```python
from build123d import *

# Parameters (mm, degrees)
F1_DEPTH = 120
F2_T     = -2
F3_W     = 48
F3_H     = 27.5
F4_DEPTH = 3


with BuildPart() as f1:
    # F0 (on Right) → F1 (new body)
    with BuildSketch(Plane.YZ):
        Polygon((0, 0), (0, 52), (-55, 52), (-94, 22), (-94, 0), align=None)
    extrude(amount=F1_DEPTH)

    # F2
    f2_openings = [f1.faces().sort_by_distance(p)[0] for p in [
        (60, -27.5, 52),
    ]]
    offset(amount=F2_T, openings=f2_openings, kind=Kind.INTERSECTION)

    # F3 (on face) → F4 (cut)
    with BuildSketch(Plane(origin=(0, -45.5762081784, 59.249070632), x_dir=(1, 0, 0), z_dir=(0, -0.6097107608, 0.7926239891))):
        with Locations((84, -41.3430182371)):
            Rectangle(F3_W, F3_H)
    extrude(amount=-F4_DEPTH, mode=Mode.SUBTRACT)


solid = f1.part
```
CAD build for the part. Positions are in the model's coordinates, mm. A direction names the side the tool comes from. Round coordinates to 2 decimals unless told otherwise and drop trailing zeros. Order: outer loops, then holes, each group sorted by start corner. A loop starts at its lowest first (then second) coordinate and runs counter-clockwise, first axis right, second up. Notation, with made-up numbers: (-6.5, 78) - (48.5, 78) arc R30 cw to (48.5, 106) - close; hole circle Ø11 at (-39.75, -6.75). An arc over 180 degrees is marked (long way). Use CSV: the item, a comma, the result in double quotes. Start each with the question number.
1) Saw through at B-B (z = 19). List the corners of the cut face in (x, y).
2) Two-plate mould, pull along X, no slides. Class faces 1 (the flat face through (46, -52, 52)), 2 (the flat face through (60, -78, 33)), 3 (the flat face through (120, -48, 26)): pulls with the +X half, pulls with the -X half, needs draft (parallel to the pull), parting line crosses it, or undercut.
3) Saw through at C-C (y = -22). List the corners of the cut face in (x, z).
4) Saw through at D-D (x = 37). List the corners of the cut face in (y, z), and give its area (3 significant figures).
5) Wall check: L1, parallel to X at y = -70, z = 39; L2, parallel to Y at x = 24.5, z = 6; L3, parallel to X at y = -22, z = 7. Give the ranges that are in metal, low to high. Write a range as [from, to].
6) Tool access for faces 4 (the flat face through (59, -92, 12)), 5 (the flat face through (59, -94, 11)), 6 (the flat face through (59, -2, 27)): list every direction of +Z, -Z, +X, -X, +Y, -Y with a clear straight run to the whole face (end or side of a thin tool).
7) Saw through at A-A (x = 68). List the corners of the cut face in (y, z).
8) Pin check, flat tips, straight feed: pin 1 Ø2 at (x, y) = (67.5, -74.5) entering from +Z; pin 2 Ø5 at (x, z) = (23.5, 29.5) entering from -Y. Stop position of each tip, or through.
Values follow:
1,outline,"(0, -94) - (120, -94) - (120, 0) - (0, 0) - close; hole (2, -92) - (118, -92) - (118, -2) - (2, -2) - close"
2,face 1,"needs draft"
2,face 2,"undercut"
2,face 3,"pulls with the +X half"
3,outline,"(0, 0) - (120, 0) - (120, 52) - (118, 52) - (118, 2) - (2, 2) - (2, 52) - (0, 52) - close"
4,outline,"(-94, 0) - (0, 0) - (0, 52) - (-2, 52) - (-2, 2) - (-92, 2) - (-92, 21.02) - (-51.72, 52) - (-55, 52) - (-94, 22) - close"
4,area,"427 mm2"
5,L1,"x = [0, 60], [108, 120]"
5,L2,"y = [-94, -92], [-2, 0]"
5,L3,"x = [0, 2], [118, 120]"
6,face 4,"none"
6,face 5,"+Z, -Z, +X, -X, -Y"
6,face 6,"+Z"
7,outline,"(-94, 0) - (0, 0) - (0, 52) - (-2, 52) - (-2, 2) - (-92, 2) - (-92, 21.02) - (-88.02, 24.07) - (-89.24, 25.66) - (-94, 22) - close; (-67.45, 42.43) - (-66.23, 40.84) - (-51.72, 52) - (-55, 52) - close"
8,pin 1,"stops at z = 2"
8,pin 2,"stops at y = -87.5"
